Source: CAD feature listing. Evaluate the final solid. Frame: model axes, mm. A direction names the side the tool comes from. Give positions to 0.01 mm unless a question says otherwise; leave off trailing zeros. Write each loop counter-clockwise with the first axis right and the second up, starting at its lowest first coordinate (ties: lowest second). Pieces come first, ordered by that corner, then holes. Notation, with made-up numbers: (10.5, 70) -> (45.5, 70) arc R28 cw to (45.5, 90) -> close; hole circle Ø1 at (77, -40). An arc over 180 degrees is marked (long way). Answer as a JSON object with one key per item and string values. Group by question number.
Item 1: Section query A-A on x = -81. Return the cut outline in (y, z).
Item 2: Section query B-B on x = -13. Return the cut outline in (y, z), plus the area to 3 significant figures.
Item 3: Section query C-C on z = 24. Return the cut outline in (x, y) (1 decimal), plus the area to 3 significant figures.
Item 4: Ray query, probe 1 along X at (y, z) = (75.5, 2) (1 decimal); probe 2 along X at (y, z) = (57, 8.25) (1 decimal); probe 3 along X at (y, z) = (-15, 6.5) (3 decimals). Return the intervals inside material, ascending. Write a range as from..to.
Item 5: Section query D-D on y = 18.5. Return the cut outline in (x, z) (1 decimal), plus the area to 3 significant figures.
Item 6: First-contact query: pin 1 Ø1.5 at (y, z) = (18, 6) entering from +X; pin 2 Ø1.7 at (x, y) = (-4.76, 71.44) entering from -Z; pin 3 Ø4 at (x, y) = (-5, 22.5) entering from +Z; pin 4 Ø10 at (x, y) = (-75, 85) entering from -Z. Flat tips, straight axial feed; report the tip coordinate or a pass-through.
Item 7: Access query for faces 1 (the face through (-96, 86.511, 3)), 2 (the face through (-12.656, 2.371, 7.617)), 3 (the face through (-5.28, 2.44, 3.15)), 4 (the face through (-18.415, 82, 5)). Directions: +Z, -Z, +X, -X, +Y, -Y. A direction counts if a zero-diameter tool reaches every point of the face in a straight line with its end or side. Return the directions, or none.
Item 8: Pull-direction query (X, two-part tool) for faces 5 (the face through (-26.035, -16, 3)), 6 (the face through (-6, 72, 4.762)); classes: pulls with the +X half, pulls with the -X half, needs draft (parallel to the pull), parting line crosses it, or undercut.
from build123d import *

# Parameters (mm, degrees)
SKETCH1_W                          = 9.525
SKETCH1_H                          = 76.2
BOSS_EXTRUDE1_DEPTH                = 1.5875
CHAMFER2_SIZE                      = 1.5875
F_97_0_0825_DIAMETER_HOLE1_D       = 2.0955
SKETCH5_R                          = 2.38125
SKETCH5_R_2                        = 1.04775
BOSS_EXTRUDE2_DEPTH                = 3.175
BOSS_EXTRUDE4_REACH                = 77.644
SKETCH7_W                          = 1.5875
SKETCH7_H                          = 75.318017262
BOSS_EXTRUDE4_DIRECTION_2_DEPTH    = 12.7
CUT_EXTRUDE1_DEPTH                 = 83.855524788
BOSS_EXTRUDE5_DEPTH                = 8.89
BOSS_EXTRUDE7_DEPTH                = 2.54
BOSS_EXTRUDE11_DEPTH               = 2.54
BOSS_EXTRUDE8_DEPTH                = 84.074
BOSS_EXTRUDE12_REACH               = 143.095
SKETCH18_W                         = 2.54
SKETCH18_H                         = 111.72801717
CUT_EXTRUDE2_DEPTH                 = 160.515381323
CUT_EXTRUDE2_DEPTH_BACK            = 2.54
SKETCH19_W                         = 61.214
SKETCH19_H                         = 12.7
SKETCH20_W                         = 10.16
SKETCH20_H                         = 10.16
BOSS_EXTRUDE13_DEPTH               = 5.08
CUT_EXTRUDE3_DEPTH                 = 128.89819871
CUT_EXTRUDE3_DEPTH_BACK            = 128.89819871
F_97_0_14_DIAMETER_HOLE1_OUTLINE_R = 1.778
F_97_0_14_DIAMETER_HOLE1_DEPTH     = 5.08
CUT_EXTRUDE4_DEPTH                 = 1.27


# Read off the part's stored shape, not the designer's step: #97 (0.14) Diameter Hole1
with BuildPart() as part:
    # Sketch1 → Boss-Extrude1 (new body)
    with BuildSketch(Plane.XY):
        with Locations((-4.7625, 38.1)):
            Rectangle(SKETCH1_W, SKETCH1_H)
    extrude(amount=BOSS_EXTRUDE1_DEPTH)

    # Chamfer2
    chamfer2_edges = [part.edges().sort_by_distance(p)[0] for p in [
        (0, 0, 0.79375),
        (-9.525, 0, 0.79375),
        (-9.525, 76.2, 0.79375),
        (0, 76.2, 0.79375),
    ]]
    chamfer(chamfer2_edges, length=CHAMFER2_SIZE)

    # #97 (0.0825) Diameter Hole1 (through all)
    with Locations(Plane.XY.offset(1.5875)):
        with Locations((-4.7625, 4.7625), (-4.7625, 71.4375)):
            Hole(F_97_0_0825_DIAMETER_HOLE1_D / 2)

    # Sketch5 → Boss-Extrude2 (add)
    # profile 1 of 2: a face of its own
    with BuildSketch(Plane.XY.offset(1.5875)):
        with Locations((-4.7625, 4.7625)):
            Circle(SKETCH5_R)
        with Locations((-4.7625, 4.7625)):
            Circle(SKETCH5_R_2, mode=Mode.SUBTRACT)
    # profile 2 of 2: a face of its own
    with BuildSketch(Plane.XY.offset(1.5875)):
        with Locations(Location((-4.7625, 71.4375, 0), (0, 0, 180))):
            Circle(SKETCH5_R)
        with Locations((-4.7625, 71.4375)):
            Circle(SKETCH5_R_2, mode=Mode.SUBTRACT)
    extrude(amount=BOSS_EXTRUDE2_DEPTH)

    # Boss-Extrude4: up to this face of the body (flat: up to its plane)
    boss_extrude4_end = Plane(part.part.faces().sort_by_distance((-4.7625, 38.1, 0))[0])
    # Sketch7 → Boss-Extrude4 (add, up to the picked face)
    with BuildSketch(Plane(origin=(0, 2.297711148, 13.030967461), x_dir=(-1, 0, 0), z_dir=(0, -0.1736481776669307, -0.984807753012208)), mode=Mode.PRIVATE) as boss_extrude4_sk1:
        with Locations((8.73125, 37.383342149)):
            Rectangle(SKETCH7_W, SKETCH7_H)
    boss_extrude4_tool1 = split(extrude(boss_extrude4_sk1.sketch, amount=BOSS_EXTRUDE4_REACH, mode=Mode.PRIVATE), bisect_by=boss_extrude4_end, keep=Keep.BOTH, mode=Mode.PRIVATE)
    add(boss_extrude4_tool1.solids().sort_by(Axis((-8.73125, 39.113116, 6.539418), (0, -0.1736481776669307, -0.984807753012208)))[0])

    # Sketch7 → Boss-Extrude4 direction 2 (add)
    with BuildSketch(Plane(origin=(0, 2.297711148, 13.030967461), x_dir=(-1, 0, 0), z_dir=(0, -0.1736481776669307, -0.984807753012208))):
        with Locations((8.73125, 37.383342149)):
            Rectangle(SKETCH7_W, SKETCH7_H)
    extrude(amount=-BOSS_EXTRUDE4_DIRECTION_2_DEPTH)

    # Sketch9 → Cut-Extrude1 (cut, through all)
    with BuildSketch(Plane(origin=(-7.9375, 0, 0), x_dir=(0, 0, -1), z_dir=(1, 0, 0))):
        Polygon((0, 0), (-1.5875, 0), (0, -0.279919082), align=None)
    extrude(amount=-CUT_EXTRUDE1_DEPTH, mode=Mode.SUBTRACT)

    # Sketch10 → Boss-Extrude5 (add)
    with BuildSketch(Plane.ZY.offset(9.525)):
        Polygon((25.585894906, 4.231564516), (12.507058463, 78.405331856), (5.002823385, 77.082132743), (5.443889757, 74.58072105), (10.446713142, 75.462853792), (22.643416842, 6.291909837), (7.39996286, 3.604077621), (7.841029232, 1.102665928), align=None)
    extrude(amount=BOSS_EXTRUDE5_DEPTH)

    # Sketch12 → Boss-Extrude7 (add)
    with BuildSketch(Plane.ZY.offset(18.415)):
        Polygon((25.144828535, 6.732976208), (29.28981052, -16.774384765), (0, -21.93896862), (0, 2.299264512), align=None)
    extrude(amount=-BOSS_EXTRUDE7_DEPTH)

    # Sketch17 → Boss-Extrude11 (add)
    with BuildSketch(Plane.ZY.offset(18.415)):
        Polygon((12.948124835, 75.903920164), (0, 73.620816406), (0, 96.671000496), (9.006311201, 98.259056157), align=None)
    extrude(amount=-BOSS_EXTRUDE11_DEPTH)

    # Sketch13 → Boss-Extrude8 (add)
    with BuildSketch(Plane.ZY.offset(18.415)):
        Polygon((9.006311201, 98.259056157), (0, 96.671000496), (0, 94.091816901), (6.94596588, 95.316578093), (26.347332456, -14.714039444), (0, -19.359785026), (0, -21.93896862), (29.28981052, -16.774384765), align=None)
    extrude(amount=BOSS_EXTRUDE8_DEPTH)

    # Boss-Extrude12: up to this plane
    boss_extrude12_end = Plane(origin=(-15.875, 2.299264512, 0), z_dir=(0, 0, -1))
    # Sketch18 → Boss-Extrude12 (add, up to the surface)
    with BuildSketch(Plane(origin=(0, 4.061976633, 23.036614231), x_dir=(-1, 0, 0), z_dir=(0, -0.17364817766693072, -0.9848077530122081)), mode=Mode.PRIVATE) as boss_extrude12_sk1:
        with Locations((101.219, 36.798342195)):
            Rectangle(SKETCH18_W, SKETCH18_H)
    boss_extrude12_tool1 = split(extrude(boss_extrude12_sk1.sketch, amount=BOSS_EXTRUDE12_REACH, mode=Mode.PRIVATE), bisect_by=boss_extrude12_end, keep=Keep.BOTH, mode=Mode.PRIVATE)
    add(boss_extrude12_tool1.solids().sort_by_distance((-101.219, 40.301269, 16.646649))[0])

    # Sketch19 → Cut-Extrude2 (cut, two sides: drawn at the far end of the back side and taken through both)
    with BuildSketch(Plane(origin=(0, -21.27742777, 3.751784596), x_dir=(-1, 0, 0), z_dir=(0, -0.984807753012208, 0.17364817766693108)).offset(-CUT_EXTRUDE2_DEPTH_BACK)):
        with Locations((59.182, -11.961991138)):
            Rectangle(SKETCH19_W, SKETCH19_H)
    extrude(amount=CUT_EXTRUDE2_DEPTH + CUT_EXTRUDE2_DEPTH_BACK, mode=Mode.SUBTRACT)

    # Sketch20 → Boss-Extrude13 (add)
    with BuildSketch(Plane(origin=(0, 0, 0), x_dir=(-1, 0, 0), z_dir=(0, 0, -1))):
        with Locations((97.409, -16.85896862)):
            Rectangle(SKETCH20_W, SKETCH20_H)
        with Locations((20.955, -16.85896862)):
            Rectangle(SKETCH20_W, SKETCH20_H)
        with Locations((20.955, 91.591000496)):
            Rectangle(SKETCH20_W, SKETCH20_H)
        with Locations((97.409, 91.591000496)):
            Rectangle(SKETCH20_W, SKETCH20_H)
    extrude(amount=-BOSS_EXTRUDE13_DEPTH)

    # Sketch21 → Cut-Extrude3 (cut, two sides: drawn at the far end of the back side and taken through both)
    with BuildSketch(Plane.ZY.offset(26.035).offset(-CUT_EXTRUDE3_DEPTH_BACK)):
        Polygon((0, -21.93896862), (5.08, -21.043227558), (5.08, -21.93896862), align=None)
    extrude(amount=CUT_EXTRUDE3_DEPTH + CUT_EXTRUDE3_DEPTH_BACK, mode=Mode.SUBTRACT)

    # #97 (0.14) Diameter Hole1 outline → #97 (0.14) Diameter Hole1 (cut)
    with BuildSketch(Plane.XY):
        with Locations((-97.409, 91.591000496)):
            Circle(F_97_0_14_DIAMETER_HOLE1_OUTLINE_R)
        with Locations((-20.955, 91.591000496)):
            Circle(F_97_0_14_DIAMETER_HOLE1_OUTLINE_R)
        with Locations((-97.409, -16.85896862)):
            Circle(F_97_0_14_DIAMETER_HOLE1_OUTLINE_R)
    extrude(amount=F_97_0_14_DIAMETER_HOLE1_DEPTH, mode=Mode.SUBTRACT)

    # 97 _0.14_ Diameter Hole1 2 outline → 97 _0.14_ Diameter Hole1 2 (revolve, cut)
    with BuildSketch(Plane(origin=(-20.955, -16.85896862, 0), x_dir=(1, 0, 0), z_dir=(0, -1, 0))):
        Polygon((0, 0), (1.778000002, 0), (1.778, 5.08), (1.584438765, 5.196303323), (0, 5.196303323), align=None)
    revolve(axis=Axis((-20.955, -16.85896862, 0), (0, 0, 1)), mode=Mode.SUBTRACT)

    # Sketch24 → Cut-Extrude4 (cut)
    with BuildSketch(Plane(origin=(-92.329, 0, 0), x_dir=(0, 0, -1), z_dir=(1, 0, 0))):
        Polygon((0, -19.359785026), (-5.08, -18.464043964), (-5.08, -11.77896862), (0, -11.77896862), align=None)
    extrude(amount=-CUT_EXTRUDE4_DEPTH, mode=Mode.SUBTRACT)


solid = part.part
Worked answers:
{
 "1": {"outline": "(-21.94, 0) -> (-19.36, 0) -> (-17.8, 8.84) -> (-20.3, 9.28) -> close; (-18.1, 21.79) -> (-15.6, 21.34) -> (-14.71, 26.35) -> (95.32, 6.95) -> (94.09, 0) -> (96.67, 0) -> (98.26, 9.01) -> (-16.77, 29.29) -> close"},
 "2": {"outline": "(1.1, 7.84) -> (3.6, 7.4) -> (6.29, 22.64) -> (75.46, 10.45) -> (74.58, 5.44) -> (77.08, 5) -> (78.41, 12.51) -> (4.23, 25.59) -> close", "area": "244 mm^2"},
 "3": {"outline": "(-102.5, -17.7) -> (-15.9, -17.7) -> (-15.9, 4) -> (-7.9, 4) -> (-7.9, 13.2) -> (-102.5, 13.2) -> close; hole (-99.9, -15.1) -> (-18.4, -15.1) -> (-18.4, -1.4) -> (-99.9, -1.4) -> close", "area": "1,630 mm^2"},
 "4": {"probe 1": "-102.5..-99.9, -18.4..-15.9, -9.5..-7.9", "probe 2": "-102.5..-99.9, -9.5..-7.9", "probe 3": "-102.489..-99.949, -18.415..-15.875"},
 "5": {"outline": "(-102.5, 0) -> (-99.9, 0) -> (-99.9, 20.5) -> (-9.5, 20.5) -> (-9.5, 0) -> (0, 0) -> (0, 1.6) -> (-7.9, 1.6) -> (-7.9, 23.1) -> (-102.5, 23.1) -> close", "area": "341 mm^2"},
 "6": {"pin 1": "x = -7.94", "pin 2": "through", "pin 3": "z = 1.59", "pin 4": "z = 7.88"},
 "7": {"face 1": "-Z", "face 2": "-Z, -Y", "face 3": "+Z", "face 4": "none"},
 "8": {"face 5": "undercut", "face 6": "needs draft"}
}
